The listing builds one solid part. Answer for the finished solid, in the listing's coordinates (mm). A direction names the side the tool comes from. Give positions to 0.01 mm unless a question says otherwise; leave off trailing zeros. Loops run counter-clockwise (first coordinate to the right, second up) from the corner with the lowest first, then second, coordinate; pieces in that order, holes last. Notation, with made-up numbers: M -33,-15.75 L -7,-15.75 A10 cw -7,-4.75 Z; hole C -25,50 d4. An arc over 180 degrees is marked long. Return JSON: item names as keys, results as strings.
from build123d import *

# Parameters (mm, degrees)
F0_W     = 32.0205967701
F0_H     = 31.4794032299
F1_DEPTH = 12.7
F2_W     = 6.35
F2_H     = 6.35
F3_DEPTH = 6.35
F5_DEPTH = 6.35


with BuildPart() as f1:
    # F0 (on Front) → F1 (new body)
    with BuildSketch(Plane.XZ):
        with Locations((-16.0102983851, 15.7397016149)):
            Rectangle(F0_W, F0_H)
        Polygon((0, 31.4794032299), (0, 0), (-32.0205967701, 0), (-32.0205967701, -32.0205967701), (31.4794032299, -32.0205967701), (31.4794032299, 31.4794032299), align=None)
    extrude(amount=F1_DEPTH)

    # F2 (on face) → F3 (join)
    with BuildSketch(Plane.XZ.offset(12.7)):
        Polygon((31.4794032299, 25.1294032299), (31.4794032299, 31.4794032299), (-25.6705967701, 31.4794032299), (-25.6705967701, 25.1294032299), (-19.3205967701, 25.1294032299), align=None)
        Polygon((-19.3205967701, -19.3205967701), (-19.3205967701, 25.1294032299), (-25.6705967701, 25.1294032299), (-25.6705967701, -25.6705967701), (-19.3205967701, -25.6705967701), align=None)
        Polygon((18.7794032299, -19.3205967701), (-19.3205967701, -19.3205967701), (-19.3205967701, -25.6705967701), (25.1294032299, -25.6705967701), (25.1294032299, -19.3205967701), align=None)
        Polygon((18.7794032299, 12.4294032299), (18.7794032299, -19.3205967701), (25.1294032299, -19.3205967701), (25.1294032299, 18.7794032299), (18.7794032299, 18.7794032299), align=None)
        Polygon((-6.6205967701, 12.4294032299), (18.7794032299, 12.4294032299), (18.7794032299, 18.7794032299), (-12.9705967701, 18.7794032299), (-12.9705967701, 12.4294032299), align=None)
        Polygon((-6.6205967701, -6.6205967701), (-6.6205967701, 12.4294032299), (-12.9705967701, 12.4294032299), (-12.9705967701, -12.9705967701), (-6.6205967701, -12.9705967701), align=None)
        Polygon((6.0794032299, -6.6205967701), (-6.6205967701, -6.6205967701), (-6.6205967701, -12.9705967701), (12.4294032299, -12.9705967701), (12.4294032299, -6.6205967701), align=None)
        Polygon((6.0794032299, -0.2705967701), (6.0794032299, -6.6205967701), (12.4294032299, -6.6205967701), (12.4294032299, 6.0794032299), (6.0794032299, 6.0794032299), align=None)
        with Locations((2.9044032299, 2.9044032299)):
            Rectangle(F2_W, F2_H)
    extrude(amount=F3_DEPTH)

    # F4 (on face) → F5 (join)
    with BuildSketch(Plane.XZ.offset(12.7)):
        Polygon((2.9044032299, 18.7794032299), (6.0794032299, 18.7794032299), (9.2544032299, 18.7794032299), (9.2544032299, 25.1294032299), (2.9044032299, 25.1294032299), align=None)
        Polygon((-12.9705967701, 2.9044032299), (-12.9705967701, 6.0794032299), (-19.3205967701, 6.0794032299), (-19.3205967701, 0), (-12.9705967701, 0), align=None)
        Polygon((-3.4455967701, -12.9705967701), (-3.4455967701, -19.3205967701), (2.8999124188, -19.3205967701), (2.8999124188, -12.9705967701), (-0.2705967701, -12.9705967701), align=None)
        Polygon((12.4294032299, -6.6205967701), (18.7794032299, -6.6205967701), (18.7794032299, -0.2705967701), (12.4294032299, -0.2705967701), (12.4294032299, -3.4455967701), align=None)
    extrude(amount=F5_DEPTH)


solid = f1.part
(1) The part is cut by section B-B (z = 8.5). Determine the outline of the cut face in (x, y).
Values follow:
{"outline": "M -32.02,-12.7 L -25.67,-12.7 L -25.67,-19.05 L -19.32,-19.05 L -19.32,-12.7 L -12.97,-12.7 L -12.97,-19.05 L -6.62,-19.05 L -6.62,-12.7 L 18.78,-12.7 L 18.78,-19.05 L 25.13,-19.05 L 25.13,-12.7 L 31.48,-12.7 L 31.48,0 L -32.02,0 Z"}
(2) The part is cut by section D-D (x = 7). Determine the outline of the cut face in (y, z), and give its area (3 significant figures).
Values follow:
{"outline": "M -19.05,-25.67 L -12.7,-25.67 L -12.7,-32.02 L 0,-32.02 L 0,31.48 L -19.05,31.48 L -19.05,12.43 L -12.7,12.43 L -12.7,6.08 L -19.05,6.08 L -19.05,-12.97 L -12.7,-12.97 L -12.7,-19.32 L -19.05,-19.32 Z", "area": "1,090 mm²"}
(3) A tool of negligible diameter and unlimited length cuts with its end or side. For faces 1 (the flat face through (0, -16, -6.621)), 2 (the flat face through (25.129, -16, -4)), 3 (the flat face through (-25.671, -16, 3)), from which of +Z, -Z, +X, -X, +Y, -Y can it reach the whole face along a straight path? Write none if from no direction.
Values follow:
{"face 1": "-Y", "face 2": "-Z, +X, -Y", "face 3": "+Z, -Z, -X, -Y"}
(4) The part is cut by section A-A (x = 20). Determine the outline of the cut face in (y, z), and give its area (3 significant figures).
Values follow:
{"outline": "M -19.05,-25.67 L -12.7,-25.67 L -12.7,-32.02 L 0,-32.02 L 0,31.48 L -19.05,31.48 L -19.05,25.13 L -12.7,25.13 L -12.7,18.78 L -19.05,18.78 Z", "area": "1,130 mm²"}
(5) Determine the mould class of faces 4 (the flat face through (0, -9, 31.479)), 5 (the flat face through (31.479, -7, -1)), 6 (the flat face through (9.254, -16, 22)) for opening direction Z: released by +Z, released by -Z, zero draft, split by the parting line, or undercut.
Values follow:
{"face 4": "released by +Z", "face 5": "zero draft", "face 6": "undercut"}
(6) Given pin 1 (3 mm diameter, centred on x = 2, z = -1, fed in from +Y); pin 2 (3 mm diameter, centred on y = -17.5, z = -16.5, fed in from +X); pin 3 (7 mm diameter, centred on x = 7.5, y = -17, fed in from -Z); pin 4 (5 mm diameter, centred on y = -16, z = -11, fed in from -X), each flat-ended and moving along its own axis, determine where each tip first touches the part or whether it passes through.
Values follow:
{"pin 1": "y = 0", "pin 2": "x = 25.13", "pin 3": "z = -25.67", "pin 4": "x = -25.67"}
(7) The part is cut by section C-C (y = -15.75). Give the number of separate pieces and of enclosed holes in the cut face, and give its area (3 significant figures).
Values follow:
{"separate pieces": "1", "enclosed holes": "4", "area": "1,970 mm²"}
(8) Straight lines are drawn through the part: line 1 along X through (y, z) = (-18, 4); line 2 along X through (y, z) = (-15.25, 8); line 3 along Z through (x, y) = (-18, -17). For each, find the intervals that lie inside material, in ascending order.
Values follow:
{"line 1": "-25.67 to -6.62, -0.27 to 12.43, 18.78 to 25.13", "line 2": "-25.67 to -19.32, -12.97 to -6.62, 18.78 to 25.13", "line 3": "-25.67 to -19.32, 0 to 6.08, 25.13 to 31.48"}
